Build history of the part. All positions in model axes, mm. A direction names the side the tool comes from. Coordinates: 2 decimals unless noted, no trailing zeros. Write each loop counter-clockwise with the first axis right and the second up, starting at its lowest first coordinate (ties: lowest second). Pieces come first, ordered by that corner, then holes. Notation, with made-up numbers: M 10.5,84.5 L 47.5,84.5 A15 cw 47.5,110.5 Z; hole C -14,79 d11. An arc over 180 degrees is marked long. Use CSV: the item, a comma, the result in double quotes. Start each with the question number.
```python
from build123d import *

# Parameters (mm, degrees)
BOSS_EXTRUDE1_DEPTH = 5
BOSS_EXTRUDE2_DEPTH = 5


with BuildPart() as part:
    # Sketch1 → Boss-Extrude1 (new body)
    with BuildSketch(Plane.XY):
        Polygon((0, 0), (8.752594228, 12.5), (0, 25), (12.5, 16.247405772), (25, 25), (16.247405772, 12.5), (25, 0), (12.5, 8.752594228), align=None)
    extrude(amount=BOSS_EXTRUDE1_DEPTH)

    # Sketch2 → Boss-Extrude2 (add)
    with BuildSketch(Plane.XY.offset(5)):
        with BuildLine():
            Line((0, 22.5), (0, 25))
            Line((0, 25), (2.5, 25))
            ThreePointArc((2.5, 25), (1.767766953, 23.232233047), (0, 22.5))
        make_face()
        with BuildLine():
            Line((25, 22.5), (25, 25))
            Line((25, 25), (22.5, 25))
            ThreePointArc((22.5, 25), (23.232233047, 23.232233047), (25, 22.5))
        make_face()
        with BuildLine():
            Line((25, 0), (22.5, 0))
            ThreePointArc((22.5, 0), (23.232233047, 1.767766953), (25, 2.5))
            Line((25, 2.5), (25, 0))
        make_face()
        with BuildLine():
            Line((0, 2.5), (0, 0))
            Line((0, 0), (2.5, 0))
            ThreePointArc((2.5, 0), (1.767766953, 1.767766953), (0, 2.5))
        make_face()
    extrude(amount=-BOSS_EXTRUDE2_DEPTH)


solid = part.part
```
1. Pull direction Y, two halves, no side cores. Call faces 1 (the flat face through (0, 24, 3)), 2 (the flat face through (24, 0, 3)), 3 (the cylindrical face through (22.6, 24.3, 2.5)), 4 (the cylindrical face through (24.24, 2.38, 2.54)): pulls with the +Y half, pulls with the -Y half, needs draft (parallel to the pull), parting line crosses it, or undercut.
2. Slice it at B-B (x = 17.5). List the corners of the cut face in (y, z).
3. Slice it at A-A (y = 20.5). List the corners of the cut face in (x, z).
4. Slice it at D-D (y = 10). List the corners of the cut face in (x, z), and give its area (3 significant figures).
5. Flat gauge pins, fed straight in: pin 1 (3 mm diameter, centred on x = 6, z = 2.5, fed in from -Y); pin 2 (3 mm diameter, centred on x = 11.5, z = 2.5, fed in from -Y). Where does each tip first touch, or does it go through?
6. 3-axis set-ups, long thin cutter, end or side, ignore diameter. For faces 5 (the cylindrical face through (2.4, 24.3, 2.5)), 6 (the flat face through (25, 24, 3)): which of +Z, -Z, +X, -X, +Y, -Y reach the whole face in a straight line?
7. Drill centre lines: line 1 along Y through (x, z) = (5.25, 0.4); line 2 along Y through (x, z) = (21, 0.95); line 3 along X through (y, z) = (20.25, 1.5). Where is each one in solid material? Low to high. Write a range as from..to.
8. Slice it at C-C (z = 1.55). List the corners of the cut face in (x, y), and give its area (3 significant figures).
Established:
1,face 1,"needs draft"
1,face 2,"pulls with the -Y half"
1,face 3,"undercut"
1,face 4,"undercut"
2,outline,"M 5.25,0 L 10.71,0 L 10.71,5 L 5.25,5 Z; M 14.29,0 L 19.75,0 L 19.75,5 L 14.29,5 Z"
3,outline,"M 3.15,0 L 6.43,0 L 6.43,5 L 3.15,5 Z; M 18.57,0 L 21.85,0 L 21.85,5 L 18.57,5 Z"
4,outline,"M 7,0 L 18,0 L 18,5 L 7,5 Z"
4,area,"55.0 mm2"
5,pin 1,"stops at y = 3.15"
5,pin 2,"stops at y = 7"
6,face 5,"+Z, -Z"
6,face 6,"+Z, -Z, +X, +Y, -Y"
7,line 1,"y = 3.68..7.5, 17.5..21.32"
7,line 2,"y = 2.8..5.71, 19.29..22.2"
7,line 3,"x = 3.33..6.78, 18.22..21.67"
8,outline,"M 0,0 L 2.5,0 A2.5 ccw 2.05,1.43 L 12.5,8.75 L 22.95,1.43 A2.5 ccw 22.5,0 L 25,0 L 25,2.5 A2.5 ccw 23.57,2.05 L 16.25,12.5 L 23.57,22.95 A2.5 ccw 25,22.5 L 25,25 L 22.5,25 A2.5 ccw 22.95,23.57 L 12.5,16.25 L 2.05,23.57 A2.5 ccw 2.5,25 L 0,25 L 0,22.5 A2.5 ccw 1.43,22.95 L 8.75,12.5 L 1.43,2.05 A2.5 ccw 0,2.5 Z"
8,area,"203 mm2"
